Check sheet for the drawn part. Datum: minimum x, y, z corner. Units: mm. A direction names the side the tool comes from. Give positions to 0.01 mm unless a question says otherwise; leave off trailing zeros. Order: outer loops, then holes, each group sorted by start corner. A loop starts at its lowest first (then second) coordinate and runs counter-clockwise, first axis right, second up. Notation, with made-up numbers: M 19,-19 L 55,-19 A12 cw 55,-15 Z; hole C 17.25,72.25 d6. An arc over 180 degrees is marked long. Answer as CSV lines item,"result". Start each with the question number.
Q1. Thickness scan on line 1 (Y direction, x = 20, z = 5.75) (3 decimals); line 2 (X direction, y = 25, z = 4.75); line 3 (Y direction, x = 21, z = 3.25) (3 decimals). Record the ranges inside material, lowest first.
Q2. Section check C-C, the plane y = 54. Record the boundary of the cut face in (x, z), then the cut area to 3 significant figures.
Q3. Go/stop test with flat-tipped pins: pin 1 (2 mm diameter, centred on x = 34.5, z = 4, fed in from +Y); pin 2 (2 mm diameter, centred on y = 37.5, z = 9, fed in from +X); pin 3 (3 mm diameter, centred on y = 25.5, z = 3, fed in from -X). Record where each tip stops, or that it passes through.
Q4. Mould release check, pull along X, two halves, no side actions. Record for the marked faces 1, 2, 3 and 4: +X half, -X half, draft (parallel to the pull), parting line (faces both ways), or undercut.
Q5. Set-up check for the marked faces 5 and 6: record each of +Z, -Z, +X, -X, +Y, -Y from which the full face is reachable in a straight line by a thin tool's end or side.
Q6. Section check A-A, the plane x = 20. Record the boundary of the cut face in (y, z) (3 decimals), then the cut area to 3 significant figures.
Q7. Section check B-B, the plane z = 5. Record the boundary of the cut face in (x, y) (1 decimal).
Q8. Section check D-D, the plane y = 20. Record the boundary of the cut face in (x, z), then the cut area to 3 significant figures.
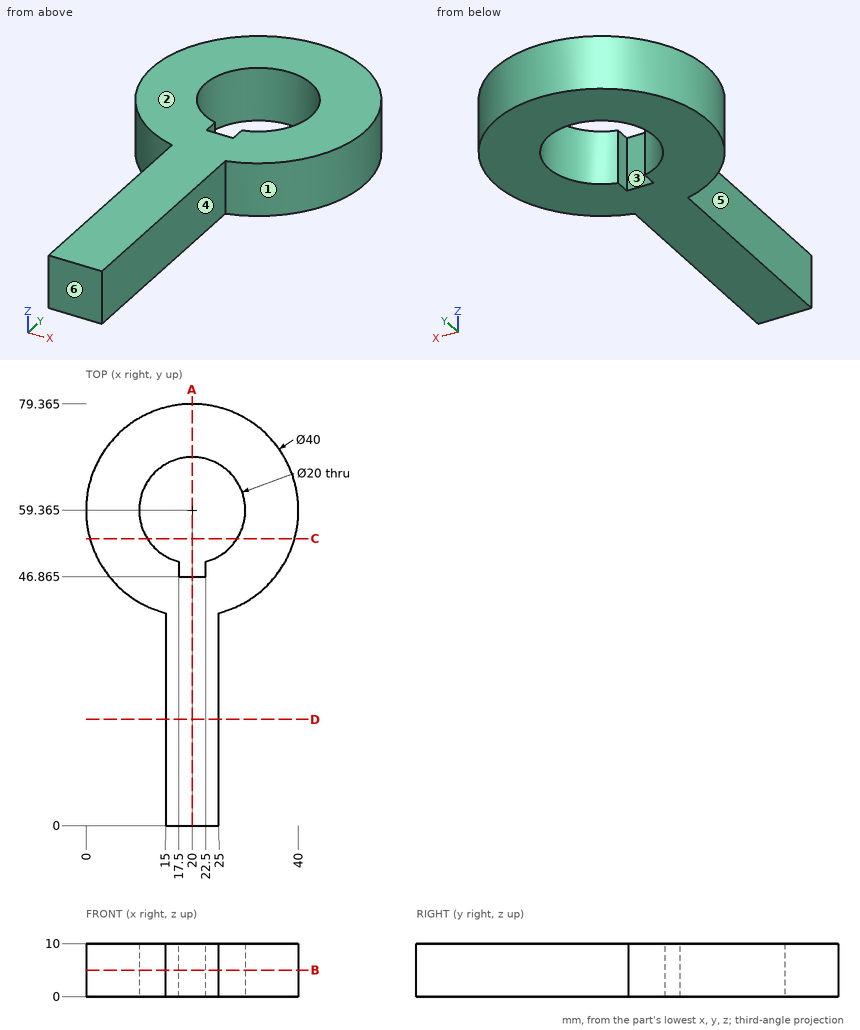
Answer block:
1,line 1,"y = 0 to 46.865, 69.365 to 79.365"
1,line 2,"x = 15 to 25"
1,line 3,"y = 0 to 46.865, 69.315 to 79.34"
2,outline,"M 0.73,0 L 11.56,0 L 11.56,10 L 0.73,10 Z; M 28.44,0 L 39.27,0 L 39.27,10 L 28.44,10 Z"
2,area,"217 mm2"
3,pin 1,"stops at y = 74.12"
3,pin 2,"stops at x = 25"
3,pin 3,"stops at x = 15"
4,face 1,"parting line"
4,face 2,"draft"
4,face 3,"undercut"
4,face 4,"+X half"
5,face 5,"+Z, -Z, -X, -Y"
5,face 6,"+Z, -Z, +X, -X, -Y"
6,outline,"M 0,0 L 46.865,0 L 46.865,10 L 0,10 Z; M 69.365,0 L 79.365,0 L 79.365,10 L 69.365,10 Z"
6,area,"569 mm2"
7,outline,"M 15,0 L 25,0 L 25,40 A20 ccw long 15,40 Z; hole M 17.5,46.9 L 22.5,46.9 L 22.5,49.7 A10 ccw long 17.5,49.7 Z"
8,outline,"M 15,0 L 25,0 L 25,10 L 15,10 Z"
8,area,"100 mm2"
